Source: CAD feature listing. Evaluate the final solid. Frame: model axes, mm. Face numbers are marked on the shaded views. Give positions to 0.01 mm unless a question says otherwise; leave off trailing zeros. Write each loop counter-clockwise with the first axis right and the second up, starting at its lowest first coordinate (ties: lowest second). Pieces come first, ordered by that corner, then holes. Notation, with made-up numbers: (1, 83) -> (32, 83) arc R13 cw to (32, 95) -> close; hole circle Ø2 at (58, 45.5). An arc over 180 degrees is marked (long way). Write item = value, one per line.
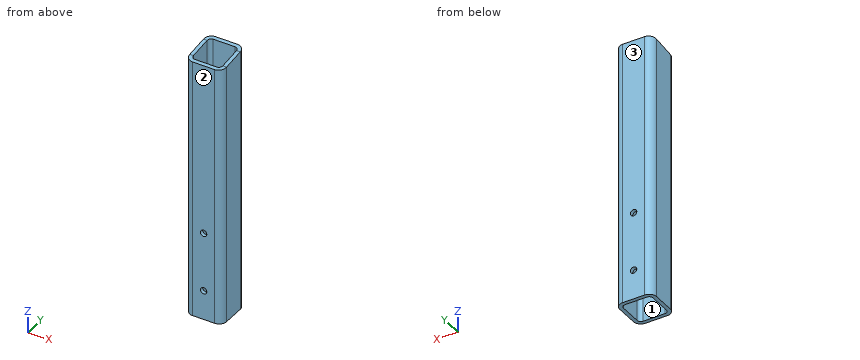
from build123d import *

# Parameters (mm, degrees)
BOSS_EXTRUDE1_DEPTH = 228.6
SKETCH3_R           = 5.55625
CUT_EXTRUDE1_DEPTH  = 64.5
CUT_EXTRUDE2_DEPTH  = 64.5


with BuildPart() as part:
    # Sketch1 → Boss-Extrude1 (new body, symmetric)
    with BuildSketch(Plane.XY):
        with BuildLine():
            Line((19.05, 31.75), (-19.05, 31.75))
            ThreePointArc((-19.05, 31.75), (-28.030256121, 28.030256121), (-31.75, 19.05))
            Line((-31.75, 19.05), (-31.75, -19.05))
            ThreePointArc((-31.75, -19.05), (-28.030256121, -28.030256121), (-19.05, -31.75))
            Line((-19.05, -31.75), (19.05, -31.75))
            ThreePointArc((19.05, -31.75), (28.030256121, -28.030256121), (31.75, -19.05))
            Line((31.75, -19.05), (31.75, 19.05))
            ThreePointArc((31.75, 19.05), (28.030256121, 28.030256121), (19.05, 31.75))
        make_face()
        with BuildLine():
            ThreePointArc((-25.4, -19.05), (-23.540128061, -23.540128061), (-19.05, -25.4))
            Line((-19.05, -25.4), (19.05, -25.4))
            ThreePointArc((19.05, -25.4), (23.540128061, -23.540128061), (25.4, -19.05))
            Line((25.4, -19.05), (25.4, 19.05))
            ThreePointArc((25.4, 19.05), (23.540128061, 23.540128061), (19.05, 25.4))
            Line((19.05, 25.4), (-19.05, 25.4))
            ThreePointArc((-19.05, 25.4), (-23.540128061, 23.540128061), (-25.4, 19.05))
            Line((-25.4, 19.05), (-25.4, -19.05))
        make_face(mode=Mode.SUBTRACT)
    extrude(amount=BOSS_EXTRUDE1_DEPTH, both=True)

    # Sketch3 → Cut-Extrude1 (cut, through all)
    with BuildSketch(Plane(origin=(0, 31.75, 0), x_dir=(1, 0, 0), z_dir=(0, 1, 0))):
        with Locations((0, 177.8)):
            Circle(SKETCH3_R)
        with Locations((0, 76.2)):
            Circle(SKETCH3_R)
    extrude(amount=-CUT_EXTRUDE1_DEPTH, mode=Mode.SUBTRACT)

    # Sketch4 → Cut-Extrude2 (cut, through all)
    with BuildSketch(Plane(origin=(31.75, 0, 0), x_dir=(0, 0, -1), z_dir=(1, 0, 0))):
        Polygon((-221.912053123, -19.05), (-228.6, -19.05), (-228.6, -114.266943845), (-209.376504653, -114.266943845), align=None)
        Polygon((-226.928013281, 19.05), (-228.6, 19.05), (-228.6, -19.05), (-221.912053123, -19.05), align=None)
        Polygon((-226.928013281, 19.05), (-228.6, 31.75), (-228.6, 19.05), align=None)
    extrude(amount=-CUT_EXTRUDE2_DEPTH, mode=Mode.SUBTRACT)


solid = part.part
1) Cut plane A-A (z = -76.2). Return the cut outline in (x, y).
Computed:
outline = (-31.75, -19.05) arc R12.7 ccw to (-19.05, -31.75) -> (-5.56, -31.75) -> (-5.56, -25.4) -> (-19.05, -25.4) arc R6.35 cw to (-25.4, -19.05) -> (-25.4, 19.05) arc R6.35 cw to (-19.05, 25.4) -> (-5.56, 25.4) -> (-5.56, 31.75) -> (-19.05, 31.75) arc R12.7 ccw to (-31.75, 19.05) -> close; (5.56, -31.75) -> (19.05, -31.75) arc R12.7 ccw to (31.75, -19.05) -> (31.75, 19.05) arc R12.7 ccw to (19.05, 31.75) -> (5.56, 31.75) -> (5.56, 25.4) -> (19.05, 25.4) arc R6.35 cw to (25.4, 19.05) -> (25.4, -19.05) arc R6.35 cw to (19.05, -25.4) -> (5.56, -25.4) -> close
2) Cut plane C-C (y = -13.5). Return the cut outline in (x, z).
Computed:
outline = (-31.75, -228.6) -> (-25.4, -228.6) -> (-25.4, 222.64) -> (-31.75, 222.64) -> close; (25.4, -228.6) -> (31.75, -228.6) -> (31.75, 222.64) -> (25.4, 222.64) -> close
3) Cut plane B-B (x = 0). Return the cut outline in (y, z).
Computed:
outline = (-31.75, -228.6) -> (-25.4, -228.6) -> (-25.4, -183.36) -> (-31.75, -183.36) -> close; (-31.75, -172.24) -> (-25.4, -172.24) -> (-25.4, -81.76) -> (-31.75, -81.76) -> close; (-31.75, -70.64) -> (-25.4, -70.64) -> (-25.4, 221.08) -> (-31.75, 220.24) -> close; (25.4, -228.6) -> (31.75, -228.6) -> (31.75, -183.36) -> (25.4, -183.36) -> close; (25.4, -172.24) -> (31.75, -172.24) -> (31.75, -81.76) -> (25.4, -81.76) -> close; (25.4, -70.64) -> (31.75, -70.64) -> (31.75, 228.6) -> (25.4, 227.76) -> close
4) Contact query for flat-ended pins moving along their axis: pin 1 (1 mm diameter, centred on y = -23, z = 144.5, fed in from +X); pin 2 (5 mm diameter, centred on x = 25, z = -165, fed in from +Y); pin 3 (18 mm diameter, centred on x = 0, z = -76.2, fed in from +Y); pin 4 (6.5 mm diameter, centred on x = 0, z = -177.8, fed in from -Y). Output: stop coordinate, or through.
Computed:
pin_1 = 31.27
pin_2 = 31.27
pin_3 = 31.75
pin_4 = through
5) Draft query along Y for the marked faces 1, 2 and 3. Return one class per face: pulls with the +Y half, pulls with the -Y half, needs draft (parallel to the pull), parting line crosses it, or undercut.
Computed:
face_1 = undercut
face_2 = pulls with the -Y half
face_3 = pulls with the +Y half
6) Cut plane D-D (z = 185). Return the cut outline in (x, y), then the cut area to 3 significant figures.
Computed:
outline = (-31.75, -19.05) arc R12.7 ccw to (-19.05, -31.75) -> (19.05, -31.75) arc R12.7 ccw to (31.75, -19.05) -> (31.75, 19.05) arc R12.7 ccw to (19.05, 31.75) -> (-19.05, 31.75) arc R12.7 ccw to (-31.75, 19.05) -> close; hole (-25.4, -19.05) arc R6.35 ccw to (-19.05, -25.4) -> (19.05, -25.4) arc R6.35 ccw to (25.4, -19.05) -> (25.4, 19.05) arc R6.35 ccw to (19.05, 25.4) -> (-19.05, 25.4) arc R6.35 ccw to (-25.4, 19.05) -> close
area = 1,350 mm²
7) Material intervals for L1, parallel to X at y = 17, z = -130.5; L2, parallel to Z at x = 0, y = -27.5, sorted ascending.
Computed:
L1 = -31.75 to -25.4, 25.4 to 31.75
L2 = -228.6 to -183.36, -172.24 to -81.76, -70.64 to 220.8
